Source: CAD feature listing. Evaluate the final solid. Frame: model axes, mm. A direction names the side the tool comes from. Coordinates: 2 decimals unless noted, no trailing zeros. Loops run counter-clockwise (first coordinate to the right, second up) from the corner with the lowest first, then second, coordinate; pieces in that order, holes last.
Item 1: Line query: probe 1 along X at (y, z) = (17, 2.4); probe 2 along Y at (x, z) = (34, 2.65); probe 3 along Y at (x, z) = (42.5, 0.2). Output: solid intervals per line, ascending.
Item 2: Pin query (flat end, axial travel): pin 1 Ø1.5 at (x, z) = (30, 1.5) entering from +Y; pin 2 Ø10.5 at (x, y) = (45.66, 13.59) entering from +Z; pin 3 Ø1.5 at (y, z) = (1, 1) entering from -X; pin 4 Ø1.5 at (x, z) = (67.5, 2.5) entering from +Y. Return the tip coordinate at first contact, or that it passes through.
Item 3: Reachability of faces 4 (the flat face through (37.292, 28.066, 1.479)), 5 (the flat face through (44.161, -1, 1)), 6 (the cylindrical face through (74.885, -30.589, 0.493)) from +Z, -Z, +X, -X, +Y, -Y: full face, straight path, thin tool, end or side. Return the list, or none.
Item 4: Section query D-D, the plane z = 0.45. State how many separate pieces and enclosed holes the cut face has, then the cut area to 3 significant figures.
Item 5: Section query C-C, the plane y = -6. Return the cut outline in (x, z), then the cut area to 3 significant figures.
Item 6: Section query A-A, the plane y = -20. Return the cut outline in (x, z), then the cut area to 3 significant figures.
Item 7: Pull-direction query (X, two-part tool) for faces 1 (the cylindrical face through (-7.52, 48.32, 1.48)), 2 (the cylindrical face through (50.865, 18.306, 1.479)), 3 (the cylindrical face through (-1, 45.89, 1.99)); classes: +X half, -X half, draft (parallel to the pull), parting line (faces both ways), or undercut.
Item 8: Section query B-B, the plane x = 61.5. Return the cut outline in (y, z), then the cut area to 3 significant figures.
Autodesk Inventor part; units mm, degrees
ref_plane "YZ Plane" through (0, 0, 0) normal (1, 0, 0) x (0, 1, 0)
ref_plane "XZ Plane" through (0, 0, 0) normal (0, 1, 0) x (-1, 0, 0)
ref_plane "XY Plane" through (0, 0, 0) normal (0, 0, 1) x (1, 0, 0)
sketch "スケッチ1" plane through (0, 0, 0) normal (0, 0, 1) x (1, 0, 0)
  circle A0 centre (-1.9226, 44.1165) radius 4
  circle A1 centre (71.1898, -32.1215) radius 4
  circle A2 centre (71.1898, -32.1215) radius 2
  circle A3 centre (-1.9226, 44.1165) radius 2
  circle A4 centre (22.3463, 32.4678) radius 2
  circle A5 centre (45.6606, 13.5882) radius 4.025
  arc A6 (1.567, 50.1847) -> (-6.9748, 39.2714) centre (-1.9226, 44.1165) ccw
  arc A7 (66.1375, -36.9666) -> (77.3028, -28.7112) centre (71.1898, -32.1215) ccw
  arc A8 (51.7955, 17.0107) -> (49.703, 19.3336) centre (45.6606, 13.5882) ccw
  arc A9 (25.2234, 36.5571) -> (24.8388, 36.8022) centre (22.3463, 32.4678) ccw
  line L0 (1.567, 50.1847) -> (24.8388, 36.8022)
  line L1 (25.2234, 36.5571) -> (49.703, 19.3336)
  line L2 (51.7955, 17.0107) -> (77.3028, -28.7112)
  line L3 (-6.9748, 39.2714) -> (66.1375, -36.9666)
  point P0 (0, 0)
  point P1 (0, 0)
  dimension "d0" = 3
  dimension "d1" = 3
  dimension "d2" = 3
  dimension "d3" = 3
extrude "押し出し1" add sketch "スケッチ1" along normal blind 3 contours A0 | A1 | L0 A9 L1 A8 L2 A7 L3 A6
extrude "押し出し2" cut sketch "スケッチ1" along normal blind 1 contours A0 | A1
sketch "スケッチ2" plane through (0, 0, 0) normal (0, 0, -1) x (-1, 0, 0)
  circle A0 centre (1.9226, 44.1165) radius 4
  circle A1 centre (-71.1898, -32.1215) radius 4
  arc A2 (-77.3028, -28.7112) -> (-66.1375, -36.9666) centre (-71.1898, -32.1215) ccw
  line L0 (6.9748, 39.2714) -> (-66.1375, -36.9666)
  arc A3 (6.9748, 39.2714) -> (-1.567, 50.1847) centre (1.9226, 44.1165) ccw
  line L1 (-24.8388, 36.8022) -> (-1.567, 50.1847)
  arc A4 (-24.8388, 36.8022) -> (-25.2234, 36.5571) centre (-22.3463, 32.4678) ccw
  line L2 (-49.703, 19.3336) -> (-25.2234, 36.5571)
  arc A5 (-49.703, 19.3336) -> (-51.7955, 17.0107) centre (-45.6606, 13.5882) ccw
  line L3 (-77.3028, -28.7112) -> (-51.7955, 17.0107)
  circle A6 centre (-22.3463, 32.4678) radius 2
  circle A7 centre (-45.6606, 13.5882) radius 4.025
  arc A8 (-23.3433, 34.2016) -> (-23.4971, 34.1035) centre (-22.3463, 32.4678) ccw
  line L4 (-23.3433, 34.2016) -> (-0.0714, 47.5841)
  arc A9 (4.8096, 41.3479) -> (-0.0714, 47.5841) centre (1.9226, 44.1165) ccw
  line L5 (4.8096, 41.3479) -> (-68.3028, -34.8902)
  arc A10 (-74.683, -30.1728) -> (-68.3028, -34.8902) centre (-71.1898, -32.1215) ccw
  line L6 (-74.683, -30.1728) -> (-49.1757, 15.5492)
  arc A11 (-47.9767, 16.8801) -> (-49.1757, 15.5492) centre (-45.6606, 13.5882) ccw
  line L7 (-47.9767, 16.8801) -> (-23.4971, 34.1035)
  circle A12 centre (1.9226, 44.1165) radius 7
  circle A13 centre (-71.1898, -32.1215) radius 7
  circle A14 centre (-45.6606, 13.5882) radius 7.025
  circle A15 centre (-22.3463, 32.4678) radius 5
  line L8 (-45.6606, 13.5882) -> (-5.0774, 13.5882) construction
  line L9 (-45.6606, 12.0882) -> (-5.0774, 12.0882)
  line L10 (-5.0774, 15.0882) -> (-45.6606, 15.0882)
  arc A16 (-45.6606, 15.0882) -> (-45.6606, 12.0882) centre (-45.6606, 13.5882) ccw
  arc A17 (-5.0774, 12.0882) -> (-5.0774, 15.0882) centre (-5.0774, 13.5882) ccw
  line L11 (-45.6606, 13.5882) -> (-45.6606, -36.9666) construction
  line L12 (-47.1606, 13.5882) -> (-47.1606, -36.9666)
  line L13 (-44.1606, -36.9666) -> (-44.1606, 13.5882)
  arc A18 (-44.1606, 13.5882) -> (-47.1606, 13.5882) centre (-45.6606, 13.5882) ccw
  arc A19 (-47.1606, -36.9666) -> (-44.1606, -36.9666) centre (-45.6606, -36.9666) ccw
  line L14 (-22.3463, 32.4678) -> (-21.0148, -7.0629) construction
  line L15 (-23.8454, 32.4173) -> (-22.514, -7.1134)
  line L16 (-19.5157, -7.0124) -> (-20.8471, 32.5183)
  arc A20 (-20.8471, 32.5183) -> (-23.8454, 32.4173) centre (-22.3463, 32.4678) ccw
  arc A21 (-22.514, -7.1134) -> (-19.5157, -7.0124) centre (-21.0148, -7.0629) ccw
  point P0 (0, 0)
  point P1 (-25.369, 13.5882)
  point P2 (-45.6606, -11.6892)
  point P3 (-38.7977, 15.0882)
  point P4 (-20.3735, 15.0882)
  point P5 (0.8334, 37.2018)
  point P6 (-5.0513, 44.7204)
  point P7 (-19.3707, 36.486)
  point P8 (-27.245, 31.4666)
  point P9 (-43.2679, 20.1931)
  point P10 (-44.1606, 6.7252)
  point P11 (-44.1606, -9.7159)
  point P12 (-23.2505, 12.0882)
  point P13 (-38.7977, 12.0882)
  point P14 (-47.1606, -12.8441)
  point P15 (-47.1606, 6.7252)
  point P16 (-51.9807, 10.5211)
  point P17 (-71.8842, -25.1561)
  point P18 (-64.3266, -30.744)
  point P19 (-21.6805, 12.7025)
  point P20 (-23.2618, 15.0882)
  point P21 (-23.6849, 27.6503)
  point P22 (-20.6866, 27.7513)
  point P23 (-20.2639, 15.2025)
  dimension "d8" = 3
  dimension "d9" = 3
  dimension "d10" = 3
  dimension "d11" = 3
  dimension "d12" = 3
  dimension "d13" = 3
  dimension "d14" = 3
  dimension "d17" = 3
extrude "押し出し3" cut sketch "スケッチ2" against normal through all contours A12 L5 L16 A15 L4 | L10 A14 L7 A15 L15 | L5 L13 A14 L9 | A14 L12 L5 A13 L6
fillet "フィレット1" radius 1 19 edges at (71.8842, -25.1561, 1.5) (64.3266, -30.744, 1.5) (47.1606, -12.8441, 1.5) (47.1606, 6.7252, 1.5) (51.9807, 10.5211, 1.5) (44.1606, 6.7252, 1.5) (44.1606, -9.7159, 1.5) (23.2505, 12.0882, 1.5) (23.2618, 15.0882, 1.5) (38.7977, 12.0882, 1.5) (38.7977, 15.0882, 1.5) (43.2679, 20.1931, 1.5) (23.6849, 27.6503, 1.5) (27.245, 31.4666, 1.5) (20.2639, 15.2025, 1.5) (20.6866, 27.7513, 1.5) (19.3707, 36.486, 1.5) (5.0513, 44.7204, 1.5) (-0.8334, 37.2018, 1.5)
sketch "スケッチ3" plane through (0, 0, 0) normal (0, 0, -1) x (-1, 0, 0)
  arc A0 (-64.8037, -29.2549) -> (-70.3207, -25.1757) centre (-71.1898, -32.1215) ccw
  arc A1 (-71.0698, -23.6962) -> (-70.3207, -25.1757) centre (-70.1965, -24.1834) ccw
  line L0 (-71.0698, -23.6962) -> (-52.797, 9.0579)
  arc A2 (-51.1432, 9.196) -> (-52.797, 9.0579) centre (-51.9237, 8.5707) ccw
  arc A3 (-51.1432, 9.196) -> (-47.8491, 6.9128) centre (-45.6606, 13.5882) ccw
  arc A4 (-47.1606, 5.9625) -> (-47.8491, 6.9128) centre (-48.1606, 5.9625) ccw
  line L1 (-47.1606, 5.9625) -> (-47.1606, -12.4421)
  arc A5 (-47.4389, -13.1343) -> (-47.1606, -12.4421) centre (-48.1606, -12.4421) ccw
  line L2 (-47.4389, -13.1343) -> (-63.1696, -29.5375)
  arc A6 (-64.8037, -29.2549) -> (-63.1696, -29.5375) centre (-63.8914, -28.8454) ccw
  line L3 (-24.296, 15.0882) -> (-38.035, 15.0882)
  arc A7 (-38.9852, 15.7767) -> (-38.035, 15.0882) centre (-38.035, 16.0882) ccw
  arc A8 (-38.9852, 15.7767) -> (-41.8628, 19.4981) centre (-45.6606, 13.5882) ccw
  arc A9 (-41.8976, 21.1572) -> (-41.8628, 19.4981) centre (-41.3222, 20.3394) ccw
  line L4 (-41.8976, 21.1572) -> (-28.3356, 30.6992)
  arc A10 (-26.8579, 30.3125) -> (-28.3356, 30.6992) centre (-27.7602, 29.8814) ccw
  arc A11 (-26.8579, 30.3125) -> (-24.2754, 27.855) centre (-22.3463, 32.4678) ccw
  arc A12 (-23.6618, 26.9661) -> (-24.2754, 27.855) centre (-24.6612, 26.9324) ccw
  line L5 (-23.6618, 26.9661) -> (-23.2966, 16.1219)
  arc A13 (-24.296, 15.0882) -> (-23.2966, 16.1219) centre (-24.296, 16.0882) ccw
  line L6 (-44.1606, -7.2284) -> (-44.1606, 5.9625)
  arc A14 (-43.4722, 6.9128) -> (-44.1606, 5.9625) centre (-43.1606, 5.9625) ccw
  arc A15 (-43.4722, 6.9128) -> (-38.9852, 11.3997) centre (-45.6606, 13.5882) ccw
  arc A16 (-38.035, 12.0882) -> (-38.9852, 11.3997) centre (-38.035, 11.0882) ccw
  line L7 (-38.035, 12.0882) -> (-25.595, 12.0882)
  arc A17 (-24.8733, 10.396) -> (-25.595, 12.0882) centre (-25.595, 11.0882) ccw
  line L8 (-24.8733, 10.396) -> (-42.4389, -7.9205)
  arc A18 (-44.1606, -7.2284) -> (-42.4389, -7.9205) centre (-43.1606, -7.2284) ccw
  line L9 (-18.2147, 37.1508) -> (-6.5004, 43.8871)
  arc A19 (-5.0114, 43.1572) -> (-6.5004, 43.8871) centre (-6.0019, 43.0202) ccw
  arc A20 (-5.0114, 43.1572) -> (-0.6744, 37.6161) centre (1.9226, 44.1165) ccw
  arc A21 (-0.3236, 35.9953) -> (-0.6744, 37.6161) centre (-1.0454, 36.6874) ccw
  line L10 (-0.3236, 35.9953) -> (-18.6225, 16.914)
  arc A22 (-20.3437, 17.5725) -> (-18.6225, 16.914) centre (-19.3443, 17.6062) ccw
  line L11 (-20.3437, 17.5725) -> (-20.6635, 27.067)
  arc A23 (-20.1111, 27.9952) -> (-20.6635, 27.067) centre (-19.6641, 27.1007) ccw
  arc A24 (-20.1111, 27.9952) -> (-18.4879, 35.6479) centre (-22.3463, 32.4678) ccw
  arc A25 (-18.2147, 37.1508) -> (-18.4879, 35.6479) centre (-17.7162, 36.2839) ccw
  circle A26 centre (1.9226, 44.1165) radius 4
  circle A27 centre (-71.1898, -32.1215) radius 4
  arc A28 (-77.3028, -28.7112) -> (-66.1375, -36.9666) centre (-71.1898, -32.1215) ccw
  line L12 (6.9748, 39.2714) -> (-66.1375, -36.9666)
  arc A29 (6.9748, 39.2714) -> (-1.567, 50.1847) centre (1.9226, 44.1165) ccw
  line L13 (-24.8388, 36.8022) -> (-1.567, 50.1847)
  arc A30 (-24.8388, 36.8022) -> (-25.2234, 36.5571) centre (-22.3463, 32.4678) ccw
  line L14 (-49.703, 19.3336) -> (-25.2234, 36.5571)
  arc A31 (-49.703, 19.3336) -> (-51.7955, 17.0107) centre (-45.6606, 13.5882) ccw
  line L15 (-77.3028, -28.7112) -> (-51.7955, 17.0107)
  circle A32 centre (-22.3463, 32.4678) radius 2
  circle A33 centre (-45.6606, 13.5882) radius 4.025
  circle A34 centre (1.9226, 44.1165) radius 2
  circle A35 centre (-71.1898, -32.1215) radius 2
  point P0 (0, 0)
properties part number "アームフレーム小"
Verdict:
1. probe 1: x = 14.38 to 18.54, 20.14 to 23.33, 39.52 to 43.53, 47.8 to 51.8
1. probe 2: y = -3.46 to 0.88, 12.09 to 15.09, 26.71 to 30.38
1. probe 3: y = -12.32 to -7.98, 7.31 to 11.1, 16.08 to 24.4
2. pin 1: stops at y = 33.72
2. pin 2: stops at z = 3
2. pin 3: stops at x = 29.01
2. pin 4: stops at y = -9.8
3. face 4: +Z, -Z, +X, +Y
3. face 5: +Z, -Z
3. face 6: -Z
4. separate pieces: 1
4. enclosed holes: 8
4. area: 1,080 mm2
5. outline: (36.44, 0) - (40.6, 0) - (40.6, 3) - (36.44, 3) - close; (44.16, 0) - (47.16, 0) - (47.16, 3) - (44.16, 3) - close; (61.2, 0) - (64.63, 0) - (64.63, 3) - (61.2, 3) - close
5. area: 31.8 mm2
6. outline: (49.87, 0) - (54.02, 0) - (54.02, 3) - (49.87, 3) - close; (69.01, 0) - (72.44, 0) - (72.44, 3) - (69.01, 3) - close
6. area: 22.8 mm2
7. face 1: parting line
7. face 2: +X half
7. face 3: undercut
8. outline: (-32.13, 0) - (-27.8, 0) - (-27.8, 3) - (-32.13, 3) - close; (-6.54, 0) - (-0.38, 0) - (-0.38, 3) - (-6.54, 3) - close
8. area: 31.5 mm2
